Solid Edge part; units mm, degrees
sketch "Sketch1" plane through (0, 0, 0) normal (0, 0, 1) x (1, 0, 0)
  line L0 (-75, -75) -> (75, -75)
  line L1 (75, -75) -> (75, 75)
  line L2 (75, 75) -> (-75, 75)
  line L3 (-75, 75) -> (-75, -75)
  dimension "D1" = 75
extrude "Ajout_matière_1" add sketch "Sketch1" along normal blind 8
sketch "Sketch2" plane through (0, 0, 0) normal (0, 0, -1) x (-1, 0, 0)
  line L0 (-75, 75) -> (-55, 75)
  line L1 (-55, 75) -> (-55, 55)
  line L2 (-55, 55) -> (-75, 55)
  line L3 (-75, 55) -> (-75, 75)
  line L4 (75, 75) -> (55, 75)
  line L5 (55, 75) -> (55, 55)
  line L6 (55, 55) -> (75, 55)
  line L7 (75, 55) -> (75, 75)
  line L8 (75, -75) -> (55, -75)
  line L9 (55, -75) -> (55, -55)
  line L10 (55, -55) -> (75, -55)
  line L11 (75, -55) -> (75, -75)
  line L12 (-75, -75) -> (-55, -75)
  line L13 (-55, -75) -> (-55, -55)
  line L14 (-55, -55) -> (-75, -55)
  line L15 (-75, -55) -> (-75, -75)
  dimension "D1" = 55
extrude "Ajout_matière_2" add sketch "Sketch2" along normal blind 55
sketch "Sketch3" plane through (65, 65, -55) normal (0, 0, -1) x (0, 1, 0)
  line L0 (-10, -10) -> (20, -10)
  line L1 (20, -10) -> (20, 20)
  line L2 (20, 20) -> (-10, 20)
  line L3 (-10, 20) -> (-10, -10)
  line L4 (-10, -120) -> (20, -120)
  line L5 (20, -120) -> (20, -150)
  line L6 (20, -150) -> (-10, -150)
  line L7 (-10, -150) -> (-10, -120)
  line L8 (-120, -120) -> (-150, -120)
  line L9 (-150, -120) -> (-150, -150)
  line L10 (-150, -150) -> (-120, -150)
  line L11 (-120, -150) -> (-120, -120)
  line L12 (-120, -10) -> (-150, -10)
  line L13 (-150, -10) -> (-150, 20)
  line L14 (-150, 20) -> (-120, 20)
  line L15 (-120, 20) -> (-120, -10)
  dimension "D1" = 20
extrude "Ajout_matière_3" add sketch "Sketch3" along normal blind 10
fillet "Congé_1" radius 5 12 edges at (85, -85, -60) (85, -55, -60) (55, -85, -60) (-85, -85, -60) (-55, -85, -60) (-85, -55, -60) (-85, 55, -60) (-85, 85, -60) (-55, 85, -60) (55, 85, -60) (85, 85, -60) (85, 55, -60)
sketch "Sketch4" plane through (0, 0, 8) normal (0, 0, 1) x (0, -1, 0)
  circle A0 centre (0, 0) radius 57.5
  circle A1 centre (0, 0) radius 45
extrude "Enlèvement_matière_1" cut sketch "Sketch4" against normal blind 3
sketch "Sketch5" plane through (0, 0, 8) normal (0, 0, 1) x (0, -1, 0)
  circle A0 centre (0, 0) radius 10
extrude "Enlèvement_matière_2" cut sketch "Sketch5" against normal blind 92.4618
chamfer "Chanfrein_1" distance 8 angle 45 8 edges at (65, 75, -55) (75, 65, -55) (-65, 75, -55) (-75, 65, -55) (-75, -65, -55) (-65, -75, -55) (65, -75, -55) (75, -65, -55)
sketch "Sketch6" plane through (0, 0, 0) normal (0, 0, -1) x (-1, 0, 0)
  circle A0 centre (0, 0) radius 17.5
  circle A1 centre (0, 0) radius 15
extrude "Ajout_matière_4" add sketch "Sketch6" along normal blind 55
properties material "Acier S235"
Design review of the part built by this model. Coordinates are the model's own, in mm. A direction names the side the tool comes from. Coordinates: 2 decimals unless noted, no trailing zeros. Order: outer loops, then holes, each group sorted by start corner. A loop starts at its lowest first (then second) coordinate and runs counter-clockwise, first axis right, second up. Notation, with made-up numbers: M 49,50 L 67,50 A35 ccw 67,86 Z; hole C -39,55 d3. An arc over 180 degrees is marked long. Use a Markdown table: item, result.
(1) Draft analysis for pull direction Y (two halves, no side actions). For faces 5 (the cylindrical face through (-84, -57, -60)), 6 (the flat face through (-66, -79, -51)), 7 (the cylindrical face through (-9.76, 2.17, 4.06)), 8 (the flat face through (55, 65, -32)), state which applies: released by +Y, released by -Y, zero draft, split by the parting line, or undercut.
Worked answers:
| item | result |
|---|---|
| face 5 | undercut |
| face 6 | released by -Y |
| face 7 | undercut |
| face 8 | zero draft |
(2) For faces 1 (the flat face through (3, -10, 0)), 2 (the flat face through (0, -75, 1)), 3 (the flat face through (0, 75, 1)), 4 (the flat face through (-65, -55, -32)), list the 3-axis set-ups (+Z, -Z, +X, -X, +Y, -Y) from which the entire face can be reached by the end or side of a thin tool; tool diameter is ignored.
Worked answers:
| item | result |
|---|---|
| face 1 | -Z |
| face 2 | +Z, +X, -X, -Y |
| face 3 | +Z, +X, -X, +Y |
| face 4 | -Z, +X, -X |
(3) Add section A-A (z = -29). Give the boundary of the cut face in (x, y), then the cut area to 3 significant figures.
Worked answers:
| item | result |
|---|---|
| outline | M -75,-75 L -55,-75 L -55,-55 L -75,-55 Z; M -75,55 L -55,55 L -55,75 L -75,75 Z; C 0,0 d35; M 55,-75 L 75,-75 L 75,-55 L 55,-55 Z; M 55,55 L 75,55 L 75,75 L 55,75 Z; hole C 0,0 d30 |
| area | 1,860 mm2 |
(4) Add section B-B (x = 0). Give the boundary of the cut face in (y, z), then the cut area to 3 significant figures.
Worked answers:
| item | result |
|---|---|
| outline | M -75,0 L -17.5,0 L -17.5,-55 L -15,-55 L -15,0 L -10,0 L -10,8 L -45,8 L -45,5 L -57.5,5 L -57.5,8 L -75,8 Z; M 10,0 L 15,0 L 15,-55 L 17.5,-55 L 17.5,0 L 75,0 L 75,8 L 57.5,8 L 57.5,5 L 45,5 L 45,8 L 10,8 Z |
| area | 1,240 mm2 |
(5) For P1, Ø5, axis at x = -55.5, z = -12.5, coming from the +Y side; P2, Ø15, axis at x = -2.5, y = -3.5, coming from the -Z side; P3, Ø1, axis at x = 61.5, z = -37.5, coming from the -Y side, all flat-tipped, find the tip position at first contact; note any pin that passes through.
Worked answers:
| item | result |
|---|---|
| P1 | stops at y = 75 |
| P2 | stops at z = 0 |
| P3 | stops at y = -75 |
(6) Wall thickness on probe 1 along X at (y, z) = (62.5, -13); probe 2 along Y at (x, z) = (0, -36): over which ranges is each line inside the solid? List them lowest first.
Worked answers:
| item | result |
|---|---|
| probe 1 | x = -75 to -55, 55 to 75 |
| probe 2 | y = -17.5 to -15, 15 to 17.5 |
(7) Add section D-D (x = 66). Give the boundary of the cut face in (y, z), then the cut area to 3 significant figures.
Worked answers:
| item | result |
|---|---|
| outline | M -85,-65 L -55,-65 L -55,0 L 55,0 L 55,-65 L 85,-65 L 85,-55 L 83,-55 L 75,-47 L 75,8 L -75,8 L -75,-47 L -83,-55 L -85,-55 Z |
| area | 4,060 mm2 |
